```python
from build123d import *

# Parameters (mm, degrees)
BOSS_EXTRUDE1_DEPTH = 5
SKETCH2_W           = 35
SKETCH2_H           = 65
CUT_EXTRUDE1_DEPTH  = 10
SKETCH4_W           = 30
SKETCH4_H           = 5
BOSS_EXTRUDE2_DEPTH = 5
SKETCH5_W           = 20
SKETCH5_H           = 5
CUT_EXTRUDE3_DEPTH  = 5
SKETCH6_R           = 2.1
CUT_EXTRUDE4_DEPTH  = 5
BOSS_EXTRUDE3_DEPTH = 5
SKETCH8_W           = 4.2
SKETCH8_H           = 5
SKETCH8_W_2         = 10
SKETCH8_H_2         = 10
CUT_EXTRUDE5_DEPTH  = 5
SKETCH10_W          = 30
SKETCH10_H          = 10
CUT_EXTRUDE7_DEPTH  = 6
SKETCH11_W          = 15
SKETCH11_H          = 5
SKETCH11_W_2        = 5.2
CUT_EXTRUDE8_DEPTH  = 6
SKETCH13_W          = 8.5
SKETCH13_H          = 65
BOSS_EXTRUDE5_DEPTH = 5
SKETCH14_R          = 5
SKETCH14_R_2        = 5.12829824
CUT_EXTRUDE9_DEPTH  = 5


with BuildPart() as part:
    # Sketch1 → Boss-Extrude1 (new body)
    with BuildSketch(Plane.XY):
        Polygon((95, -5), (95, 0), (115, 0), (115, 20), (120, 20), (120, 45), (115, 45), (115, 65), (100, 65), (100, 70), (70, 70), (70, 65), (-70, 65), (-70, 70), (-100, 70), (-100, 65), (-115, 65), (-115, 45), (-120, 45), (-120, 20), (-115, 20), (-115, 0), (-95, 0), (-95, -5), (-35, -5), (-35, 0), (35, 0), (35, -5), align=None)
    extrude(amount=BOSS_EXTRUDE1_DEPTH)

    # Sketch2 → Cut-Extrude1 (cut)
    with BuildSketch(Plane(origin=(0, 0, 0), x_dir=(-1, 0, 0), z_dir=(0, 0, -1))):
        with Locations((102.5, 27.5)):
            Rectangle(SKETCH2_W, SKETCH2_H)
        with Locations((-102.5, 27.5)):
            Rectangle(SKETCH2_W, SKETCH2_H)
    extrude(amount=-CUT_EXTRUDE1_DEPTH, mode=Mode.SUBTRACT)

    # Sketch4 → Boss-Extrude2 (add)
    with BuildSketch(Plane(origin=(0, 65, 0), x_dir=(1, 0, 0), z_dir=(0, 1, 0))):
        with Locations((0, -2.5)):
            Rectangle(SKETCH4_W, SKETCH4_H)
    extrude(amount=BOSS_EXTRUDE2_DEPTH)

    # Sketch5 → Cut-Extrude3 (cut)
    with BuildSketch(Plane(origin=(0, 0, 0), x_dir=(-1, 0, 0), z_dir=(0, 0, -1))):
        with Locations((-69.8, -2.5)):
            Rectangle(SKETCH5_W, SKETCH5_H)
        with Locations((69.8, -2.5)):
            Rectangle(SKETCH5_W, SKETCH5_H)
    extrude(amount=-CUT_EXTRUDE3_DEPTH, mode=Mode.SUBTRACT)

    # Sketch6 → Cut-Extrude4 (cut)
    with BuildSketch(Plane(origin=(0, 0, 0), x_dir=(-1, 0, 0), z_dir=(0, 0, -1))):
        with Locations((0, 67.5)):
            Circle(SKETCH6_R)
    extrude(amount=-CUT_EXTRUDE4_DEPTH, mode=Mode.SUBTRACT)

    # Sketch7 → Boss-Extrude3 (add)
    with BuildSketch(Plane(origin=(0, 0, 0), x_dir=(-1, 0, 0), z_dir=(0, 0, -1))):
        with BuildLine():
            Line((4.330127019, 70), (-4.330127019, 70))
            ThreePointArc((-4.330127019, 70), (0, 72.5), (4.330127019, 70))
        make_face()
    extrude(amount=-BOSS_EXTRUDE3_DEPTH)

    # Sketch8 → Cut-Extrude5 (cut)
    with BuildSketch(Plane(origin=(0, 0, 0), x_dir=(-1, 0, 0), z_dir=(0, 0, -1))):
        with Locations((69.8, 2.5)):
            Rectangle(SKETCH8_W, SKETCH8_H)
        with Locations((69.8, 10)):
            Rectangle(SKETCH8_W_2, SKETCH8_H_2)
        with Locations((-69.8, 10)):
            Rectangle(SKETCH8_W_2, SKETCH8_H_2)
        with Locations((-69.8, 2.5)):
            Rectangle(SKETCH8_W, SKETCH8_H)
        with Locations((0, 2.5)):
            Rectangle(SKETCH8_W, SKETCH8_H)
        with Locations((0, 10)):
            Rectangle(SKETCH8_W_2, SKETCH8_H_2)
    extrude(amount=-CUT_EXTRUDE5_DEPTH, mode=Mode.SUBTRACT)

    # Sketch10 → Cut-Extrude7 (cut, through all)
    with BuildSketch(Plane(origin=(0, 0, 0), x_dir=(-1, 0, 0), z_dir=(0, 0, -1))):
        with Locations((-100, 65)):
            Rectangle(SKETCH10_W, SKETCH10_H)
        with Locations((100, 65)):
            Rectangle(SKETCH10_W, SKETCH10_H)
    extrude(amount=-CUT_EXTRUDE7_DEPTH, mode=Mode.SUBTRACT)

    # Sketch11 → Cut-Extrude8 (cut, through all)
    with BuildSketch(Plane(origin=(0, 0, 0), x_dir=(-1, 0, 0), z_dir=(0, 0, -1))):
        with Locations((-77.5, 67.5)):
            Rectangle(SKETCH11_W, SKETCH11_H)
        with Locations((77.5, 67.5)):
            Rectangle(SKETCH11_W, SKETCH11_H)
        with Locations((82.4, -2.5)):
            Rectangle(SKETCH11_W_2, SKETCH11_H)
        with Locations((-82.4, -2.5)):
            Rectangle(SKETCH11_W_2, SKETCH11_H)
    extrude(amount=-CUT_EXTRUDE8_DEPTH, mode=Mode.SUBTRACT)

    # Sketch13 → Boss-Extrude5 (add)
    with BuildSketch(Plane(origin=(0, 0, 0), x_dir=(-1, 0, 0), z_dir=(0, 0, -1))):
        with Locations((-89.25, 32.5)):
            Rectangle(SKETCH13_W, SKETCH13_H)
        with Locations((89.25, 32.5)):
            Rectangle(SKETCH13_W, SKETCH13_H)
    extrude(amount=-BOSS_EXTRUDE5_DEPTH)

    # Sketch14 → Cut-Extrude9 (cut)
    with BuildSketch(Plane(origin=(0, 0, 0), x_dir=(-1, 0, 0), z_dir=(0, 0, -1))):
        with Locations((-48.915063509, 67.5)):
            Circle(SKETCH14_R)
        with Locations((48.915063509, 67.5)):
            Circle(SKETCH14_R_2)
    extrude(amount=-CUT_EXTRUDE9_DEPTH, mode=Mode.SUBTRACT)


solid = part.part
```
Source: CAD feature listing. Evaluate the final solid. Frame: model axes, mm. A direction names the side the tool comes from. Coordinates: 2 decimals unless noted, no trailing zeros. Loops run counter-clockwise (first coordinate to the right, second up) from the corner with the lowest first, then second, coordinate; pieces in that order, holes last. Notation, with made-up numbers: M 14.5,-35 L 41.5,-35 A25 cw 41.5,-18 Z; hole C 72.5,22 d10. An arc over 180 degrees is marked long. Put each result on its own line as item: value. Start each with the question number.
1) Cut plane C-C on y = 11. Return the cut outline in (x, z), then the cut area to 3 significant figures.
2) Cut plane A-A on y = 67.5. Return the cut outline in (x, z), then the cut area to 3 significant figures.
3) Pull-direction query (X, two-part tool) for faces 1 (the face through (-59.8, -3, 2)), 2 (the face through (47, -5, 2)), 3 (the face through (-64.8, 10, 2)); classes: pulls with the +X half, pulls with the -X half, needs draft (parallel to the pull), parting line crosses it, or undercut.
4) Cut plane D-D on x = 80.5. Return the cut outline in (y, z).
5) Reachability of faces 4 (the face through (-73, 65, 2)), 5 (the face through (-5, 10, 2)), 6 (the face through (18, 0, 2)), 7 (the face through (10, 70, 2)) from +Z, -Z, +X, -X, +Y, -Y: full face, straight path, thin tool, end or side. Return the list, or none.
6) Ray query, L1, parallel to X at y = 4.5, z = 4.05; L2, parallel to Y at x = 0, z = 3.4; L3, parallel to Y at x = 28.5, z = 4.4. Return the intervals inside material, ascending. Write a range as from..to.
7) Contact query for flat-ended pins moving along their axis: pin 1 Ø1.5 at (x, z) = (40, 1.5) entering from +Y; pin 2 Ø1.5 at (x, z) = (-70.5, 2) entering from -Y; pin 3 Ø1.5 at (y, z) = (-3, 2.5) entering from -X; pin 4 Ø6 at (x, y) = (26.5, 15) entering from -Z. Output: stop coordinate, or through.
8) Cut plane B-B on x = 0. Return the cut outline in (y, z), then the cut area to 4 significant figures.
The answers:
1. outline: M -93.5,0 L -74.8,0 L -74.8,5 L -93.5,5 Z; M -64.8,0 L -5,0 L -5,5 L -64.8,5 Z; M 5,0 L 64.8,0 L 64.8,5 L 5,5 Z; M 74.8,0 L 93.5,0 L 93.5,5 L 74.8,5 Z
1. area: 785 mm²
2. outline: M -15,0 L -2.1,0 L -2.1,5 L -15,5 Z; M 2.1,0 L 15,0 L 15,5 L 2.1,5 Z
2. area: 129 mm²
3. face 1: pulls with the -X half
3. face 2: needs draft
3. face 3: undercut
4. outline: M 0,0 L 65,0 L 65,5 L 0,5 Z
5. face 4: +Z, -Z, -X, +Y
5. face 5: +Z, -Z
5. face 6: +Z, -Z, -Y
5. face 7: +Z, -Z, +X, +Y
6. L1: x = -93.5..-71.9, -67.7..-2.1, 2.1..67.7, 71.9..93.5
6. L2: y = 15..65.4, 69.6..72.5
6. L3: y = 0..65
7. pin 1: stops at y = 65
7. pin 2: stops at y = 15
7. pin 3: stops at x = -59.8
7. pin 4: stops at z = 0
8. outline: M 15,0 L 65.4,0 L 65.4,5 L 15,5 Z; M 69.6,0 L 72.5,0 L 72.5,5 L 69.6,5 Z
8. area: 266.5 mm²
